from build123d import *

# Parameters (mm, degrees)
SKETCH1_W                 = 254
SKETCH1_H                 = 173.355
BOSS_EXTRUDE1_DEPTH       = 4.7625
SKETCH2_W                 = 190.5
SKETCH2_H                 = 114.3
CUT_EXTRUDE1_DEPTH        = 4.7625
BOSS_EXTRUDE2_DEPTH       = 4.7625
F_6_CLEARANCE_HOLE1_D     = 3.7973
F_6_CLEARANCE_HOLE1_DEPTH = 25.4
F_6_CLEARANCE_HOLE1_TIP   = 1.140824014
CHAMFER1_SIZE             = 2.54


with BuildPart() as part:
    # Sketch1 → Boss-Extrude1 (new body)
    with BuildSketch(Plane(origin=(0, 0, 0), x_dir=(1, 0, 0), z_dir=(0, 1, 0))):
        with Locations((127, -86.6775)):
            Rectangle(SKETCH1_W, SKETCH1_H)
    extrude(amount=BOSS_EXTRUDE1_DEPTH)

    # Sketch2 → Cut-Extrude1 (cut)
    with BuildSketch(Plane(origin=(0, 4.7625, 0), x_dir=(1, 0, 0), z_dir=(0, 1, 0))):
        with Locations((127, -86.6775)):
            Rectangle(SKETCH2_W, SKETCH2_H)
    extrude(amount=-CUT_EXTRUDE1_DEPTH, mode=Mode.SUBTRACT)

    # Sketch3 → Boss-Extrude2 (add)
    with BuildSketch(Plane(origin=(0, 4.7625, 0), x_dir=(1, 0, 0), z_dir=(0, 1, 0))):
        with BuildLine():
            Line((163.957, -29.5275), (147.447, -29.5275))
            Line((147.447, -29.5275), (147.447, -44.7675))
            ThreePointArc((147.447, -44.7675), (155.702, -53.0225), (163.957, -44.7675))
            Line((163.957, -44.7675), (163.957, -29.5275))
        make_face()
        with BuildLine():
            Line((71.247, -29.5275), (71.247, -44.7675))
            ThreePointArc((71.247, -44.7675), (79.502, -53.0225), (87.757, -44.7675))
            Line((87.757, -44.7675), (87.757, -29.5275))
            Line((87.757, -29.5275), (71.247, -29.5275))
        make_face()
        with BuildLine():
            Line((71.247, -143.8275), (87.757, -143.8275))
            Line((87.757, -143.8275), (87.757, -131.6355))
            ThreePointArc((87.757, -131.6355), (79.502, -123.3805), (71.247, -131.6355))
            Line((71.247, -131.6355), (71.247, -143.8275))
        make_face()
        with BuildLine():
            Line((147.447, -131.6355), (147.447, -143.8275))
            Line((147.447, -143.8275), (163.957, -143.8275))
            Line((163.957, -143.8275), (163.957, -131.6355))
            ThreePointArc((163.957, -131.6355), (155.702, -123.3805), (147.447, -131.6355))
        make_face()
    extrude(amount=-BOSS_EXTRUDE2_DEPTH)

    # #6 Clearance Hole1
    with Locations(Plane(origin=(0, 4.7625, 0), x_dir=(-1, 0, 0), z_dir=(0, 1, 0))):
        with Locations((-79.502, 44.7675), (-155.702, 44.7675), (-79.502, 131.6355), (-155.702, 131.6355)):
            Hole(F_6_CLEARANCE_HOLE1_D / 2, depth=F_6_CLEARANCE_HOLE1_DEPTH)
            with Locations((0, 0, -(F_6_CLEARANCE_HOLE1_DEPTH + F_6_CLEARANCE_HOLE1_TIP / 2))):  # 118° drill point
                Cone(0, F_6_CLEARANCE_HOLE1_D / 2, F_6_CLEARANCE_HOLE1_TIP, mode=Mode.SUBTRACT)

    # Chamfer1
    chamfer1_edges = [part.edges().sort_by_distance(p)[0] for p in [
        (31.75, 2.38125, 143.8275),
        (31.75, 2.38125, 29.5275),
        (222.25, 2.38125, 29.5275),
        (222.25, 2.38125, 143.8275),
        (147.447, 2.38125, 29.5275),
        (163.957, 2.38125, 29.5275),
        (71.247, 2.38125, 29.5275),
        (87.757, 2.38125, 29.5275),
        (87.757, 2.38125, 143.8275),
        (71.247, 2.38125, 143.8275),
        (163.957, 2.38125, 143.8275),
        (147.447, 2.38125, 143.8275),
    ]]
    chamfer(chamfer1_edges, length=CHAMFER1_SIZE)


solid = part.part
Can you work these out from the model? Positions are in its coordinate system, mm. A direction names the side the tool comes from. Give positions to 0.01 mm unless a question says otherwise; leave off trailing zeros. Loops run counter-clockwise (first coordinate to the right, second up) from the corner with the lowest first, then second, coordinate; pieces in that order, holes last. Notation, with made-up numbers: M 51,63.25 L 95,63.25 A16 ccw 95,94.25 Z; hole C 52,28 d9. An arc over 180 degrees is marked long. One line per item, written item: value. Start each with the question number.
1) On a 3-axis mill with a long thin cutter (end or side, diameter ignored), from which of +Z, -Z, +X, -X, +Y, -Y can I reach the whole of each face in a straight line? I mean faces 1 (the face through (0, 2, 88)), 2 (the face through (222.25, 2, 87)). Say none if no direction works.
2) Thinking about a two-plate mould opening in X: for faces 3 (the face through (153, 4.762, 47)), 4 (the face through (87.757, 2, 39)), 5 (the face through (254, 2, 88)), which applies, +X half, -X half, draft (parallel to the pull), parting line (faces both ways), or undercut?
3) If we section it at B-B, the plane z = 95: Write out the boundary of the cut face in (x, y), and give its area (3 significant figures).
4) If we section it at A-A, the plane x = 140: Write out the boundary of the cut face in (y, z) (1 decimal).
5) If we section it at C-C, the plane y = 3.8: Give the number of separate pieces and of enclosed holes in the cut face, and give its area (3 significant figures).
6) I'm going to push a flat-ended pin straight in: pin 1 (3.5 mm diameter, centred on x = 79.5, z = 44.77, fed in from +Y). Where does the tip first touch, or does it pass through?
7) If I drill on line 1 (X direction, y = 4.3, z = 131.5); line 2 (X direction, y = 4.1, z = 121.5); line 3 (Z direction, x = 101, y = 2.4) (1 decimal), over which ranges is the centre line in solid material (lowest first)? Write a range as [from, to].
Completed:
1. face 1: +Z, -Z, -X, +Y, -Y
1. face 2: +Y, -Y
2. face 3: draft
2. face 4: undercut
2. face 5: +X half
3. outline: M 0,0 L 31.75,0 L 31.75,4.76 L 0,4.76 Z; M 222.25,0 L 254,0 L 254,4.76 L 222.25,4.76 Z
3. area: 302 mm^2
4. outline: M 0,0 L 4.8,0 L 4.8,29.5 L 0,29.5 Z; M 0,143.8 L 4.8,143.8 L 4.8,173.4 L 0,173.4 Z
5. separate pieces: 1
5. enclosed holes: 5
5. area: 23,600 mm^2
6. pin 1: passes through
7. line 1: x = [0, 31.75], [71.25, 77.61], [81.4, 87.76], [147.45, 153.81], [157.6, 163.96], [222.25, 254]
7. line 2: x = [0, 31.75], [222.25, 254]
7. line 3: z = [0, 29.5], [143.8, 173.4]
